Autodesk Inventor part; units mm, degrees
ref_plane "YZ Plane" through (0, 0, 0) normal (1, 0, 0) x (0, 1, 0)
ref_plane "XZ Plane" through (0, 0, 0) normal (0, 1, 0) x (-1, 0, 0)
ref_plane "XY Plane" through (0, 0, 0) normal (0, 0, 1) x (1, 0, 0)
sketch "Skizze_1" plane through (0, 0, 0) normal (0, 0, 1) x (1, 0, 0)
  line L0 (4, 0) -> (0, 0)
  line L1 (0, 0) -> (0, 7.0725)
  line L2 (0, 7.0725) -> (2.3925, 7.0725)
  line L3 (2.3925, 7.0725) -> (4, 4.5)
  line L4 (4, 4.5) -> (4, 0)
  line L5 (4, 0) -> (0, 0)
revolve "Revolution1" add sketch "Skizze_1" angle 360 about axis through (4, 0, 0) along (1, 0, 0)
sketch "Skizze_2" plane through (0, 0, 0) normal (0, 0, 1) x (1, 0, 0)
  line L0 (4, 0) -> (0, 0)
  line L1 (0, 0) -> (0, 2)
  line L2 (0, 2) -> (0.379, 1.621)
  line L3 (0.379, 1.621) -> (3.621, 1.621)
  line L4 (3.621, 1.621) -> (4, 2)
  line L5 (4, 2) -> (4, 0)
  line L6 (4, 0) -> (0, 0)
revolve "Revolution2" cut sketch "Skizze_2" angle 360 about axis through (4, 0, 0) along (1, 0, 0)
thread "Thread1"
sketch "Skizze_3" plane through (0, 0, 0) normal (1, 0, 0) x (0, 1, 0)
  line L0 (10, 10) -> (-10, 10)
  line L1 (-10, 10) -> (-10, -10)
  line L2 (-10, -10) -> (10, -10)
  line L3 (10, -10) -> (10, 10)
  line L4 (5, 5) -> (-5, 5)
  line L5 (-5, 5) -> (-5, -5)
  line L6 (-5, -5) -> (5, -5)
  line L7 (5, -5) -> (5, 5)
extrude "Extrusion1" cut sketch "Skizze_3" along normal blind 4
properties part number "25.50.0540"
Input: part model. Units: mm. Frame: model coordinates. Round coordinates to 2 decimals unless told otherwise and drop trailing zeros. Loops run counter-clockwise (first coordinate to the right, second up) from the corner with the lowest first, then second, coordinate; pieces in that order, holes last.
1) Section query D-D on x = 3.45. Return the cut outline in (y, z), plus the area to 3 significant figures.
Ans:
outline: (-5, -1.99) arc R5.38 ccw to (-1.99, -5) - (1.99, -5) arc R5.38 ccw to (5, -1.99) - (5, 1.99) arc R5.38 ccw to (1.99, 5) - (-1.99, 5) arc R5.38 ccw to (-5, 1.99) - close; hole circle Ø3.24 at (0, 0)
area: 78.6 mm2
2) Section query A-A on y = 0. Return the cut outline in (x, z), plus the area to 3 significant figures.
Ans:
outline: (0, -5) - (3.69, -5) - (4, -4.5) - (4, -2) - (3.62, -1.62) - (0.38, -1.62) - (0, -2) - close; (0, 2) - (0.38, 1.62) - (3.62, 1.62) - (4, 2) - (4, 4.5) - (3.69, 5) - (0, 5) - close
area: 26.6 mm2
3) Pull-direction query (Y, two-part tool) for faces 1 (the cylindrical face through (2.023, 0.748, -1.438)), 2 (the flat face through (2, -5, 0)), 3 (the flat face through (2, 0, 5)); classes: released by +Y, released by -Y, zero draft, split by the parting line, or undercut.
Ans:
face 1: undercut
face 2: released by -Y
face 3: zero draft
4) Section query C-C on x = 1. Return the cut outline in (y, z), plus the area to 3 significant figures.
Ans:
outline: (-5, -5) - (5, -5) - (5, 5) - (-5, 5) - close; hole circle Ø3.24 at (0, 0)
area: 91.7 mm2
5) Material intervals for line 1 (Z direction, x = 1.6, y = 0); line 2 (Y direction, x = 1.45, z = 1); line 3 (Z direction, x = 3.3, y = 0.5), sorted ascending.
Ans:
line 1: z = -5 to -1.62, 1.62 to 5
line 2: y = -5 to -1.28, 1.28 to 5
line 3: z = -5 to -1.54, 1.54 to 5
